Check sheet for the modelled part. Datum: model origin and axes. Units: mm. Face numbers are marked on the shaded views. Give positions to 0.01 mm unless a question says otherwise; leave off trailing zeros. Write each loop counter-clockwise with the first axis right and the second up, starting at its lowest first coordinate (ties: lowest second). Pieces come first, ordered by that corner, then holes. Notation, with made-up numbers: (42.25, 24.5) -> (67.25, 24.5) arc R19 cw to (67.25, 58.5) -> close; hole circle Ø6 at (65, -33). An arc over 180 degrees is marked (long way). Answer as a JSON object with one key per item and string values.
from build123d import *

# Parameters (mm, degrees)
BASE_EXTRUSION_DEPTH    = 8
ESQUISSE2_R             = 4
ENL_V_MAT_EXTRU_1_DEPTH = 39.48376281
ESQUISSE3_R             = 4
ENL_V_MAT_EXTRU_2_DEPTH = 37.545825061
CHANFREIN1_SIZE         = 0.5


with BuildPart() as part:
    # Esquisse1 → Base-Extrusion (new body)
    with BuildSketch(Plane.XY):
        with BuildLine():
            Line((-11, 0), (-11, -25))
            ThreePointArc((-11, -25), (0, -36), (11, -25))
            Line((11, -25), (11, 0))
            ThreePointArc((11, 0), (0, 11), (-11, 0))
        make_face()
    extrude(amount=BASE_EXTRUSION_DEPTH)

    # Esquisse2 → Enlèv. mat.-Extru.1 (cut, through all)
    with BuildSketch(Plane.XY.offset(8)):
        Circle(ESQUISSE2_R)
    extrude(amount=-ENL_V_MAT_EXTRU_1_DEPTH, mode=Mode.SUBTRACT)

    # Esquisse3 → Enlèv. mat.-Extru.2 (cut, through all)
    with BuildSketch(Plane(origin=(-1.490572535, -22.400343219, 8), x_dir=(1, 0, 0), z_dir=(0, 0, 1))):
        with Locations((1.490572535, -2.599656781)):
            Circle(ESQUISSE3_R)
    extrude(amount=-ENL_V_MAT_EXTRU_2_DEPTH, mode=Mode.SUBTRACT)

    # Chanfrein1
    chanfrein1_edges = [part.edges().sort_by_distance(p)[0] for p in [
        (-4, 0, 0),
        (-4, 0, 8),
        (-4, -25, 0),
        (-4, -25, 8),
    ]]
    chamfer(chanfrein1_edges, length=CHANFREIN1_SIZE)


solid = part.part
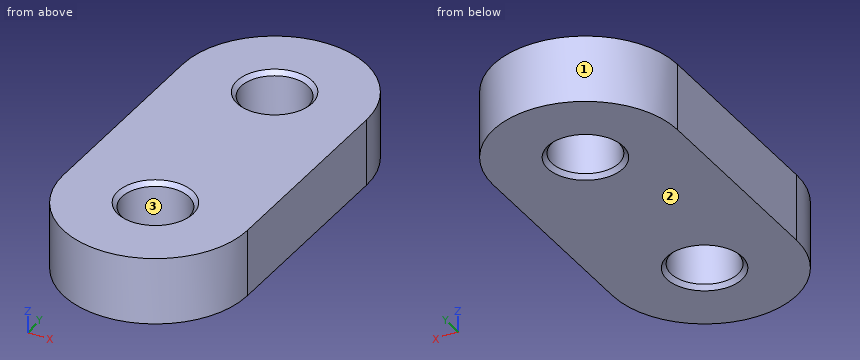
1. Sectioned sample at A-A, the plane x = 0. Enter the section's corners in (y, z).
Determined:
{"outline": "(-36, 0) -> (-29.5, 0) -> (-29, 0.5) -> (-29, 7.5) -> (-29.5, 8) -> (-36, 8) -> close; (-21, 0.5) -> (-20.5, 0) -> (-4.5, 0) -> (-4, 0.5) -> (-4, 7.5) -> (-4.5, 8) -> (-20.5, 8) -> (-21, 7.5) -> close; (4, 0.5) -> (4.5, 0) -> (11, 0) -> (11, 8) -> (4.5, 8) -> (4, 7.5) -> close"}
2. Go/stop test with flat-tipped pins: P1, Ø7, axis at x = 0, y = -25, coming from the -Z side; P2, Ø1.5, axis at x = 7.5, z = 3, coming from the -Y side; P3, Ø3, axis at x = -8, z = 4, coming from the -Y side. Record where each tip stops, or that it passes through.
Determined:
{"P1": "through", "P2": "y = -33.69", "P3": "y = -33.87"}
3. Mould release check, pull along X, two halves, no side actions. Record for the marked faces 1, 2 and 3: released by +X, released by -X, zero draft, split by the parting line, or undercut.
Determined:
{"face 1": "split by the parting line", "face 2": "zero draft", "face 3": "undercut"}
4. Sectioned sample at B-B, the plane z = 2. Enter the section's corners in (x, y), plus the area to 3 significant figures.
Determined:
{"outline": "(-11, -25) arc R11 ccw to (11, -25) -> (11, 0) arc R11 ccw to (-11, 0) -> close; hole circle Ø8 at (0, -25); hole circle Ø8 at (0, 0)", "area": "830 mm^2"}
5. Sectioned sample at C-C, the plane y = -30.5. Enter the section's corners in (x, z), plus the area to 3 significant figures.
Determined:
{"outline": "(-9.53, 0) -> (9.53, 0) -> (9.53, 8) -> (-9.53, 8) -> close", "area": "152 mm^2"}
6. Sectioned sample at D-D, the plane x = -9. Enter the section's corners in (y, z).
Determined:
{"outline": "(-31.32, 0) -> (6.32, 0) -> (6.32, 8) -> (-31.32, 8) -> close"}
7. Scan lines: L1, parallel to Y at x = 0, z = 2.5; L2, parallel to X at y = -24.5, z = 1; L3, parallel to Y at x = 1, z = 1.75. Record each from-to range of solid material in increasing order. Write a range as [from, to].
Determined:
{"L1": "[-36, -29], [-21, -4], [4, 11]", "L2": "[-11, -3.97], [3.97, 11]", "L3": "[-35.95, -28.87], [-21.13, -3.87], [3.87, 10.95]"}
